```python
from build123d import *

# Parameters (mm, degrees)
SKETCH1_R               = 7.62
SKETCH1_R_2             = 3.96875
TOP_HEAD_DEPTH          = 9.525
LOWER_START             = 6.35
SKETCH1_4_R             = 3.96875
LOWER_PIN_DEPTH         = 41.275
SKETCH2_R               = 3.175
SKETCH2_R_2             = 1.5875
O_RING_OPENING_DEPTH    = 4.7625
SKETCH2_3_R             = 1.5875
POT_SHAFT_OPENING_DEPTH = 13.589


with BuildPart() as part:
    # Sketch1 → Top Head (new body)
    # profile 1 of 2: a face of its own
    with BuildSketch(Plane.XY):
        with Locations(Location((0, 0, 0), (0, 0, 180))):
            Circle(SKETCH1_R)
        Circle(SKETCH1_R_2, mode=Mode.SUBTRACT)
    # profile 2 of 2: a face of its own
    with BuildSketch(Plane.XY):
        Circle(SKETCH1_R_2)
    extrude(amount=TOP_HEAD_DEPTH)

    # Sketch1_4 → Lower Pin (add)
    with BuildSketch(Plane.XY.offset(LOWER_START)):
        Circle(SKETCH1_4_R)
    extrude(amount=LOWER_PIN_DEPTH)

    # Sketch2 → O-Ring Opening (cut)
    # profile 1 of 2: a face of its own
    with BuildSketch(Plane(origin=(0, 0, 0), x_dir=(-1, 0, 0), z_dir=(0, 0, -1))):
        Circle(SKETCH2_R)
        Circle(SKETCH2_R_2, mode=Mode.SUBTRACT)
    # profile 2 of 2: a face of its own
    with BuildSketch(Plane(origin=(0, 0, 0), x_dir=(-1, 0, 0), z_dir=(0, 0, -1))):
        Circle(SKETCH2_R_2)
    extrude(amount=-O_RING_OPENING_DEPTH, mode=Mode.SUBTRACT)

    # Sketch2_3 → POT Shaft Opening (cut)
    with BuildSketch(Plane(origin=(0, 0, 0), x_dir=(-1, 0, 0), z_dir=(0, 0, -1))):
        Circle(SKETCH2_3_R)
    extrude(amount=-POT_SHAFT_OPENING_DEPTH, mode=Mode.SUBTRACT)


solid = part.part
```
For this review, take the finished solid that the model builds, in its own axes (mm). A direction names the side the tool comes from. Coordinates: 2 decimals unless noted, no trailing zeros. Order: outer loops, then holes, each group sorted by start corner. A loop starts at its lowest first (then second) coordinate and runs counter-clockwise, first axis right, second up. Notation, with made-up numbers: (21, 35.5) - (79, 35.5) arc R17 ccw to (79, 39.5) - close; hole circle Ø4 at (-0.75, 80.5). An arc over 180 degrees is marked (long way). Answer as a JSON object with one key per item and string values. Group by question number.
1. For faces 1 (the flat face through (-1.4, -1.4, 4.762)), 2 (the flat face through (-3, 3, 9.525)), 3 (the cylindrical face through (0.992, -7.555, 4.696)), list the 3-axis set-ups (+Z, -Z, +X, -X, +Y, -Y) from which the entire face can be reached by the end or side of a thin tool; tool diameter is ignored.
2. We need section D-D on z = 31. State the section outline as (x, y) points.
3. Clearance check with flat-ended pins moving along their axes: P1, Ø1.5, axis at y = -2.5, z = 29.5, coming from the -X side; P2, Ø2.5, axis at x = -0.5, y = 0, coming from the -Z side; P3, Ø1, axis at y = 4, z = 17.5, coming from the +X side. State where each tip first meets the part, or that it passes through.
4. For probe 1 along Y at (x, z) = (0, 10); probe 2 along Z at (x, y) = (5.25, 3.5) (3 decimals); probe 3 along Y at (x, z) = (0, 9.25), list the stretches that pass through material, from the lowest coordinate up.
5. The part is to be moulded in two halves that separate along X. For faces 4 (the cylindrical face through (-0.86, -3.874, 28.308)), 5 (the flat face through (0, 0, 47.625)), 6 (the cylindrical face through (0.69, -3.1, 2.35)), say which applies: pulls with the +X half, pulls with the -X half, needs draft (parallel to the pull), parting line crosses it, or undercut.
6. We need section C-C on z = 12. State the section outline as (x, y) points (1 decimal).
7. We need section A-A on x = 0. State the section outline as (y, z) points (1 decimal), then the cut area to 3 significant figures.
Final values:
{
 "1": {"face 1": "-Z", "face 2": "+Z", "face 3": "+Z, -Z"},
 "2": {"outline": "circle Ø7.94 at (0, 0)"},
 "3": {"P1": "x = -3.56", "P2": "z = 4.76", "P3": "x = 1.87"},
 "4": {"probe 1": "-3.97 to -1.59, 1.59 to 3.97", "probe 2": "0 to 9.525", "probe 3": "-7.62 to -1.59, 1.59 to 7.62"},
 "5": {"face 4": "parting line crosses it", "face 5": "needs draft", "face 6": "undercut"},
 "6": {"outline": "circle Ø7.9 at (0, 0); hole circle Ø3.2 at (0, 0)"},
 "7": {"outline": "(-7.6, 0) - (-3.2, 0) - (-3.2, 4.8) - (-1.6, 4.8) - (-1.6, 13.6) - (1.6, 13.6) - (1.6, 4.8) - (3.2, 4.8) - (3.2, 0) - (7.6, 0) - (7.6, 9.5) - (4, 9.5) - (4, 47.6) - (-4, 47.6) - (-4, 9.5) - (-7.6, 9.5) - close", "area": "389 mm²"}
}
